Part model, mm, in its own coordinate system. Face numbers are marked on the shaded views. Round coordinates to 2 decimals unless told otherwise and drop trailing zeros. Order: outer loops, then holes, each group sorted by start corner. A loop starts at its lowest first (then second) coordinate and runs counter-clockwise, first axis right, second up. Notation, with made-up numbers: (-37.75, -6) -> (-11.75, -6) arc R13 ccw to (-11.75, 10) -> close; hole circle Ø3 at (-12.75, 3). An arc over 180 degrees is marked (long way). Answer as a JSON object with one key per item and string values. Group by question number.
```python
from build123d import *

# Parameters (mm, degrees)
SKETCH1_R           = 4.4
SKETCH1_R_2         = 20
BOSS_EXTRUDE1_DEPTH = 15


with BuildPart() as part:
    # Sketch1 → Boss-Extrude1 (new body)
    with BuildSketch(Plane.XY):
        with BuildLine():
            Line((-50, 45), (50, 45))
            ThreePointArc((50, 45), (57.071067812, 42.071067812), (60, 35))
            Line((60, 35), (60, -35))
            ThreePointArc((60, -35), (57.071067812, -42.071067812), (50, -45))
            Line((50, -45), (-50, -45))
            ThreePointArc((-50, -45), (-57.071067812, -42.071067812), (-60, -35))
            Line((-60, -35), (-60, 35))
            ThreePointArc((-60, 35), (-57.071067812, 42.071067812), (-50, 45))
        make_face()
        with Locations((-27.5, 22.5)):
            Circle(SKETCH1_R, mode=Mode.SUBTRACT)
        with Locations((27.5, 22.5)):
            Circle(SKETCH1_R, mode=Mode.SUBTRACT)
        with Locations((-27.5, -22.5)):
            Circle(SKETCH1_R, mode=Mode.SUBTRACT)
        with Locations((27.5, -22.5)):
            Circle(SKETCH1_R, mode=Mode.SUBTRACT)
        Circle(SKETCH1_R_2, mode=Mode.SUBTRACT)
    extrude(amount=BOSS_EXTRUDE1_DEPTH)


solid = part.part
```
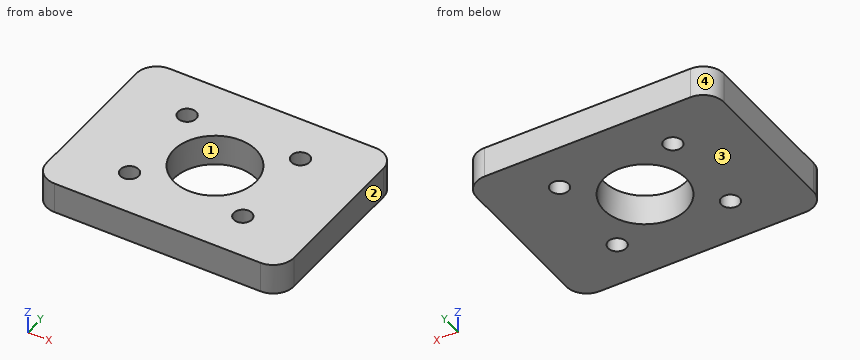
Q1. Band-saw the part on B-B (y = 0). List the corners of the cut face in (x, z), plus the area to 3 significant figures.
Q2. Band-saw the part on A-A (x = 0). List the corners of the cut face in (y, z).
Q3. Two-plate mould, pull along X, no slides. Class the marked faces 1, 2, 3 and 4: +X half, -X half, draft (parallel to the pull), parting line (faces both ways), or undercut.
Q4. Band-saw the part on C-C (y = -22.5). List the corners of the cut face in (x, z).
Q5. Band-saw the part on D-D (x = -27.5). List the corners of the cut face in (y, z), plus the area to 3 significant figures.
Q6. Wall check: line 1 (Y direction, x = 27.5, z = 10.5); line 2 (X direction, y = -18.5, z = 11.5); line 3 (Y direction, x = -30.5, z = 10.5). Give the ranges that are in metal, low to high. Write a range as [from, to].
Completed:
{
 "1": {"outline": "(-60, 0) -> (-20, 0) -> (-20, 15) -> (-60, 15) -> close; (20, 0) -> (60, 0) -> (60, 15) -> (20, 15) -> close", "area": "1,200 mm2"},
 "2": {"outline": "(-45, 0) -> (-20, 0) -> (-20, 15) -> (-45, 15) -> close; (20, 0) -> (45, 0) -> (45, 15) -> (20, 15) -> close"},
 "3": {"face 1": "undercut", "face 2": "+X half", "face 3": "draft", "face 4": "-X half"},
 "4": {"outline": "(-60, 0) -> (-31.9, 0) -> (-31.9, 15) -> (-60, 15) -> close; (-23.1, 0) -> (23.1, 0) -> (23.1, 15) -> (-23.1, 15) -> close; (31.9, 0) -> (60, 0) -> (60, 15) -> (31.9, 15) -> close"},
 "5": {"outline": "(-45, 0) -> (-26.9, 0) -> (-26.9, 15) -> (-45, 15) -> close; (-18.1, 0) -> (18.1, 0) -> (18.1, 15) -> (-18.1, 15) -> close; (26.9, 0) -> (45, 0) -> (45, 15) -> (26.9, 15) -> close", "area": "1,090 mm2"},
 "6": {"line 1": "[-45, -26.9], [-18.1, 18.1], [26.9, 45]", "line 2": "[-60, -29.33], [-25.67, -7.6], [7.6, 25.67], [29.33, 60]", "line 3": "[-45, -25.72], [-19.28, 19.28], [25.72, 45]"}
}
